Input: dimensioned drawing with shaded views. Units: mm. Origin: part minimum x, y, z. Give positions to 0.01 mm unless a question says otherwise; leave off trailing zeros. Loops run counter-clockwise (first coordinate to the right, second up) from the corner with the lowest first, then second, coordinate; pieces in that order, holes last. Notation, with made-up numbers: (38.5, -1) -> (63.5, -1) arc R28 ccw to (63.5, 33) -> close; hole circle Ø5 at (16.5, -9.5). An arc over 180 degrees is marked (long way). Answer as a JSON object with one key per item and string values.
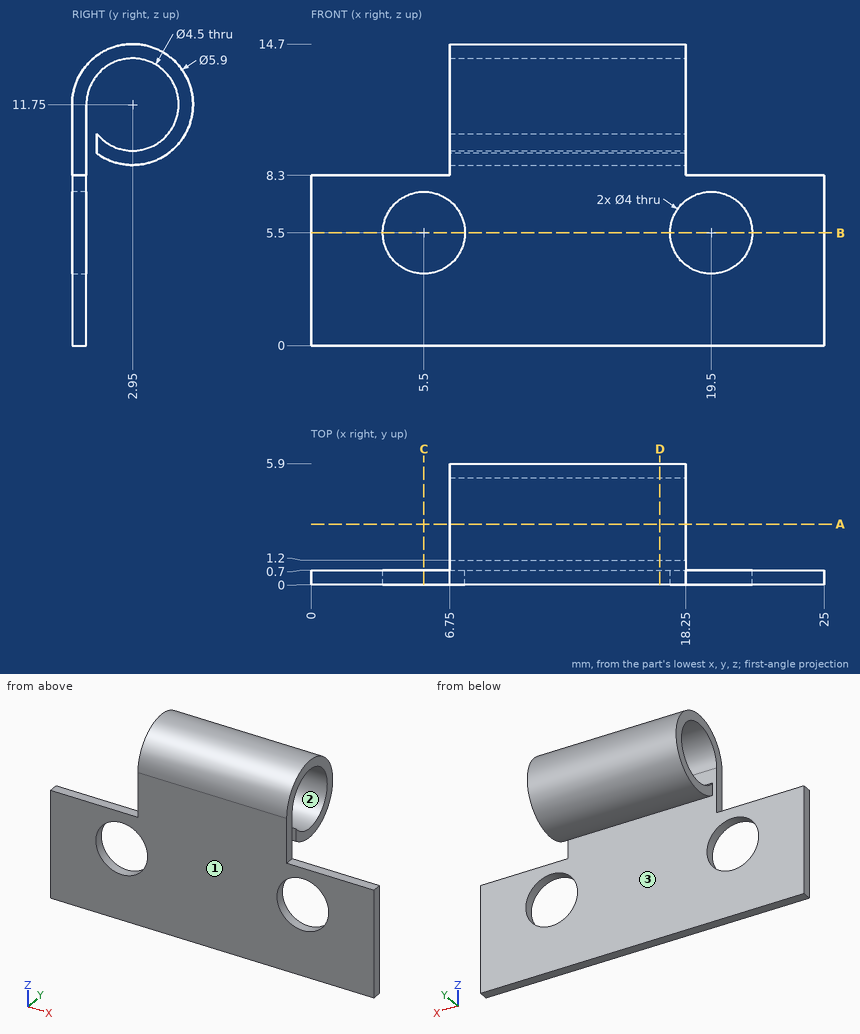
Q1. Ray query, line 1 along X through (y, z) = (0.3, 5.5); line 2 along Z through (x, y) = (13.25, 2.95); line 3 along Y through (x, z) = (10, 7). Return the intervals inside material, ascending.
Evaluation:
{"line 1": "x = 0 to 3.5, 7.5 to 17.5, 21.5 to 25", "line 2": "z = 8.8 to 9.5, 14 to 14.7", "line 3": "y = 0 to 0.7"}
Q2. Section A-A, the plane y = 2.95. Return the cut outline in (x, z).
Evaluation:
{"outline": "(6.75, 8.8) -> (18.25, 8.8) -> (18.25, 9.5) -> (6.75, 9.5) -> close; (6.75, 14) -> (18.25, 14) -> (18.25, 14.7) -> (6.75, 14.7) -> close"}
Q3. Draft query along Y for the marked faces 1, 2 and 3. Return one class per face: +Y half, -Y half, draft (parallel to the pull), parting line (faces both ways), or undercut.
Evaluation:
{"face 1": "-Y half", "face 2": "undercut", "face 3": "undercut"}
Q4. Pin query (flat end, axial travel): pin 1 (1.8 mm diameter, centred on y = 4, z = 13, fed in from -X); pin 2 (8 mm diameter, centred on x = 13, z = 12, fed in from -Y); pin 3 (3.5 mm diameter, centred on x = 9, z = 4, fed in from +Y); pin 4 (0.8 mm diameter, centred on x = 2.5, y = 0.5, fed in from +Z). Return the tip coordinate at first contact, or that it passes through.
Evaluation:
{"pin 1": "stops at x = 6.75", "pin 2": "stops at y = 0", "pin 3": "stops at y = 0.7", "pin 4": "stops at z = 8.3"}
Q5. Section C-C, the plane x = 5.5. Return the cut outline in (y, z), then the cut area to 3 significant figures.
Evaluation:
{"outline": "(0, 0) -> (0.7, 0) -> (0.7, 3.5) -> (0, 3.5) -> close; (0, 7.5) -> (0.7, 7.5) -> (0.7, 8.3) -> (0, 8.3) -> close", "area": "3.01 mm2"}
Q6. Section D-D, the plane x = 17. Return the cut outline in (y, z).
Evaluation:
{"outline": "(0, 0) -> (0.7, 0) -> (0.7, 11.75) arc R2.25 cw (long way) to (1.2, 10.34) -> (1.2, 9.38) arc R2.95 ccw (long way) to (0, 11.75) -> close"}
Q7. Section B-B, the plane z = 5.5. Return the cut outline in (x, y), then the cut area to 3 significant figures.
Evaluation:
{"outline": "(0, 0) -> (3.5, 0) -> (3.5, 0.7) -> (0, 0.7) -> close; (7.5, 0) -> (17.5, 0) -> (17.5, 0.7) -> (7.5, 0.7) -> close; (21.5, 0) -> (25, 0) -> (25, 0.7) -> (21.5, 0.7) -> close", "area": "11.9 mm2"}
